from build123d import *

# Parameters (mm, degrees)
BOSS_EXTRUDE1_DEPTH = 3
SKETCH3_W           = 9.37333333
SKETCH3_H           = 9.75
BOSS_EXTRUDE2_DEPTH = 4
SKETCH5_W           = 28.87333333
SKETCH5_H           = 21.46504359
BOSS_EXTRUDE3_DEPTH = 3
SKETCH6_R           = 1.7
CUT_EXTRUDE1_DEPTH  = 10


with BuildPart() as part:
    # Sketch1 → Boss-Extrude1 (new body)
    with BuildSketch(Plane.XY):
        Polygon((-4.686666665, 8.42561874), (-14.436666665, 8.42561874), (-14.436666665, -30.57438126), (-14.436666665, -45.57438126), (-7.270097193, -45.57438126), (-7.270097193, -30.57438126), (6.249902807, -30.57438126), (6.249902807, -45.57438126), (14.436666665, -45.57438126), (14.436666665, -30.57438126), (14.436666665, 8.42561874), (4.686666665, 8.42561874), (4.686666665, 18.17561874), (-4.686666665, 18.17561874), align=None)
    extrude(amount=BOSS_EXTRUDE1_DEPTH)

    # Sketch3 → Boss-Extrude2 (add)
    with BuildSketch(Plane.XY.offset(3)):
        with Locations((0, 13.30061874)):
            Rectangle(SKETCH3_W, SKETCH3_H)
    extrude(amount=BOSS_EXTRUDE2_DEPTH)

    # Sketch5 → Boss-Extrude3 (add)
    with BuildSketch(Plane.XY):
        with Locations((0, -34.841859465)):
            Rectangle(SKETCH5_W, SKETCH5_H)
    extrude(amount=-BOSS_EXTRUDE3_DEPTH)

    # Sketch6 → Cut-Extrude1 (cut)
    with BuildSketch(Plane.ZY.offset(4.686666665)):
        with Locations(Location((3.6, 14.31561874, 0), (0, 0, 270))):
            Circle(SKETCH6_R)
    extrude(amount=-CUT_EXTRUDE1_DEPTH, mode=Mode.SUBTRACT)


solid = part.part
Input: part model. Units: mm. Frame: model coordinates. A direction names the side the tool comes from. Give positions to 0.01 mm unless a question says otherwise; leave off trailing zeros. Write each loop counter-clockwise with the first axis right and the second up, starting at its lowest first coordinate (ties: lowest second). Pieces come first, ordered by that corner, then holes.
Q1. Section C-C, the plane x = 9.5. Output: boundary loops of the cut face in (y, z).
Q2. First-contact query: P1, Ø0.9, axis at x = 11.5, z = 1.5, coming from the +Y side; P2, Ø1.5, axis at x = 2.5, z = 1, coming from the -Y side; P3, Ø0.9, axis at x = -4, z = -1, coming from the +Y side; P4, Ø3, axis at y = 14.32, z = 3.6, coming from the -X side. Flat tips, straight axial feed; report the tip coordinate or a pass-through.
Q3. Section B-B, the plane y = -35.5. Output: boundary loops of the cut face in (x, z), plus the area to 3 significant figures.
Q4. Set-up query: faces 1 (the face through (6.25, -38, 1)), 2 (the face through (-9, 8.426, 1)), 3 (the face through (0, 8.426, 5)). Return all of +Z, -Z, +X, -X, +Y, -Y with unobstructed straight access to the full face (end or side cutting, diameter ignored); none if empty.
Q5. Material intervals for probe 1 along Z at (x, y) = (-13, -9.5); probe 2 along Y at (x, z) = (-6.75, 1); probe 3 along X at (y, z) = (13.5, 0.5), sorted ascending.
Q6. Pull-direction query (Y, two-part tool) for faces 4 (the face through (0, 18.176, 3)), 5 (the face through (0, -18, 3)), 6 (the face through (-0.066, 12.694, 4.111)), 7 (the face through (0, -45.574, -1)); classes: pulls with the +Y half, pulls with the -Y half, needs draft (parallel to the pull), parting line crosses it, or undercut.
Q7. Section D-D, the plane z = 6.25. Output: boundary loops of the cut face in (x, y), plus the area to 3 significant figures.
Q8. Section A-A, the plane z = 3.6. Output: boundary loops of the cut face in (x, y), plus the area to 3 significant figures.
Filled in:
1. outline: (-45.57, -3) - (-24.11, -3) - (-24.11, 0) - (8.43, 0) - (8.43, 3) - (-45.57, 3) - close
2. P1: stops at y = 8.43
2. P2: stops at y = -30.57
2. P3: stops at y = -24.11
2. P4: passes through
3. outline: (-14.44, -3) - (14.44, -3) - (14.44, 3) - (6.25, 3) - (6.25, 0) - (-7.27, 0) - (-7.27, 3) - (-14.44, 3) - close
3. area: 133 mm2
4. face 1: +Z, -Y
4. face 2: +Z, -Z, -X, +Y
4. face 3: +Z, +X, -X, -Y
5. probe 1: z = 0 to 3
5. probe 2: y = -30.57 to 8.43
5. probe 3: x = -4.69 to 4.69
6. face 4: pulls with the +Y half
6. face 5: needs draft
6. face 6: undercut
6. face 7: pulls with the -Y half
7. outline: (-4.69, 8.43) - (4.69, 8.43) - (4.69, 18.18) - (-4.69, 18.18) - close
7. area: 91.4 mm2
8. outline: (-4.69, 8.43) - (4.69, 8.43) - (4.69, 12.62) - (-4.69, 12.62) - close; (-4.69, 16.02) - (4.69, 16.02) - (4.69, 18.18) - (-4.69, 18.18) - close
8. area: 59.5 mm2
